from build123d import *

# Parameters (mm, degrees)
BOSS_EXTRUDE1_DEPTH     = 1.5
BOSS_EXTRUDE2_DEPTH     = 280
SKETCH4_W               = 410
SKETCH4_H               = 42.385541564
BOSS_EXTRUDE3_DEPTH     = 30
CUT_EXTRUDE1_DEPTH      = 597.860327045
CUT_EXTRUDE1_DEPTH_BACK = 597.860327045
SKETCH8_R               = 4.39
SKETCH8_R_2             = 2.39
BOSS_EXTRUDE5_DEPTH     = 15
SKETCH10_R              = 3
CUT_EXTRUDE2_DEPTH      = 1.5
SKETCH15_W              = 15
SKETCH15_H              = 1.5
SKETCH15_W_2            = 20
BOSS_EXTRUDE6_DEPTH     = 13
BOSS_EXTRUDE7_DEPTH     = 1.5
BOSS_EXTRUDE8_DEPTH     = 1.5
SKETCH20_R              = 2.415919743
SKETCH20_R_2            = 2
CUT_EXTRUDE5_DEPTH      = 1.5
SKETCH5_R               = 2
SKETCH5_R_2             = 10
CUT_EXTRUDE7_DEPTH      = 1.5
SKETCH21_W              = 300
SKETCH21_H              = 1.5
BOSS_EXTRUDE9_DEPTH     = 10
SKETCH22_W              = 300
SKETCH22_H              = 1.5
BOSS_EXTRUDE10_DEPTH    = 10
BOSS_EXTRUDE11_DEPTH    = 0.75
BOSS_EXTRUDE12_DEPTH    = 0.75
BOSS_EXTRUDE13_DEPTH    = 0.75
BOSS_EXTRUDE14_DEPTH    = 0.75
SKETCH27_W              = 200
SKETCH27_H              = 1.5
BOSS_EXTRUDE15_DEPTH    = 10
BOSS_EXTRUDE16_DEPTH    = 0.75
BOSS_EXTRUDE17_DEPTH    = 0.75
SKETCH30_R              = 24
SKETCH30_R_2            = 1.5
CUT_EXTRUDE8_DEPTH      = 1.5
SKETCH33_R              = 2
CUT_EXTRUDE9_DEPTH      = 1.5


with BuildPart() as part:
    # Sketch1 → Boss-Extrude1 (new body)
    with BuildSketch(Plane(origin=(0, 0, 0), x_dir=(1, 0, 0), z_dir=(0, 1, 0))):
        Polygon((-205, 300), (205, 300), (205, -230), (155, -230), (155, -300), (-205, -300), align=None)
    extrude(amount=BOSS_EXTRUDE1_DEPTH)

    # Sketch2 → Boss-Extrude2 (add)
    with BuildSketch(Plane(origin=(0, 1.5, 0), x_dir=(1, 0, 0), z_dir=(0, 1, 0))):
        Polygon((-205, 300), (-205, -300), (155, -300), (155, -230), (205, -230), (205, 300), align=None)
        Polygon((-203.5, 298.5), (-203.5, -298.5), (153.5, -298.5), (153.5, -228.5), (203.5, -228.5), (203.5, 298.5), align=None, mode=Mode.SUBTRACT)
    extrude(amount=BOSS_EXTRUDE2_DEPTH)

    # Sketch4 → Boss-Extrude3 (add)
    with BuildSketch(Plane(origin=(0, 0, -300), x_dir=(-1, 0, 0), z_dir=(0, 0, -1))):
        with Locations((0, 213.483316708)):
            Rectangle(SKETCH4_W, SKETCH4_H)
    extrude(amount=BOSS_EXTRUDE3_DEPTH)

    # Sketch3 → Cut-Extrude1 (cut, two sides: drawn at the far end of the back side and taken through both)
    with BuildSketch(Plane.ZY.offset(205).offset(-CUT_EXTRUDE1_DEPTH_BACK)):
        Polygon((300, 121.117558148), (228.195222706, 281.5), (300, 281.5), align=None)
    extrude(amount=CUT_EXTRUDE1_DEPTH + CUT_EXTRUDE1_DEPTH_BACK, mode=Mode.SUBTRACT)

    # Sketch8 → Boss-Extrude5 (add)
    # profile 1 of 2: a face of its own
    with BuildSketch(Plane(origin=(-203.5, 0, 0), x_dir=(0, 0, -1), z_dir=(1, 0, 0))):
        with Locations((-261.240414508, 161.097837233)):
            Circle(SKETCH8_R)
        with Locations((-261.240414508, 161.097837233)):
            Circle(SKETCH8_R_2, mode=Mode.SUBTRACT)
    # profile 2 of 2: a face of its own
    with BuildSketch(Plane(origin=(-203.5, 0, 0), x_dir=(0, 0, -1), z_dir=(1, 0, 0))):
        with Locations((-203.5, 16.5)):
            Circle(SKETCH8_R)
        with Locations((-203.5, 16.5)):
            Circle(SKETCH8_R_2, mode=Mode.SUBTRACT)
    extrude(amount=BOSS_EXTRUDE5_DEPTH)

    # Sketch10 → Cut-Extrude2 (cut)
    with BuildSketch(Plane.ZY.offset(-153.5)):
        with BuildLine():
            Line((272.25, 90.5), (258.25, 90.5))
            Line((258.25, 90.5), (258.25, 87.5))
            Line((258.25, 87.5), (254, 87.5))
            ThreePointArc((254, 87.5), (243, 76.5), (254, 65.5))
            Line((254, 65.5), (276.5, 65.5))
            ThreePointArc((276.5, 65.5), (287.5, 76.5), (276.5, 87.5))
            Line((276.5, 87.5), (272.25, 87.5))
            Line((272.25, 87.5), (272.25, 90.5))
        make_face()
        with Locations((239.3, 103.45)):
            Circle(SKETCH10_R)
        with Locations((291.2, 103.45)):
            Circle(SKETCH10_R)
        with Locations((239.3, 49.55)):
            Circle(SKETCH10_R)
        with Locations((291.2, 49.55)):
            Circle(SKETCH10_R)
    extrude(amount=-CUT_EXTRUDE2_DEPTH, mode=Mode.SUBTRACT)

    # Sketch15 → Boss-Extrude6 (add)
    with BuildSketch(Plane.ZY.offset(-203.5)):
        with Locations((-206, 251.386283415)):
            Rectangle(SKETCH15_W, SKETCH15_H)
        with Locations((74.5, 251.386283415)):
            Rectangle(SKETCH15_W_2, SKETCH15_H)
    extrude(amount=BOSS_EXTRUDE6_DEPTH)

    # Sketch17 → Boss-Extrude7 (add)
    with BuildSketch(Plane.XY.offset(-198.5)):
        Polygon((203.5, 250.636283415), (203.5, 235.636283415), (190.5, 250.636283415), align=None)
    extrude(amount=-BOSS_EXTRUDE7_DEPTH)

    # Sketch18 → Boss-Extrude8 (add)
    with BuildSketch(Plane.XY.offset(64.5)):
        Polygon((203.5, 250.636283415), (203.5, 235.636283415), (190.5, 250.636283415), align=None)
    extrude(amount=BOSS_EXTRUDE8_DEPTH)

    # Sketch20 → Cut-Extrude5 (cut)
    with BuildSketch(Plane(origin=(0, 252.136283415, 0), x_dir=(1, 0, 0), z_dir=(0, 1, 0))):
        with Locations(Location((198, 206.5, 0), (0, 0, 270))):
            Circle(SKETCH20_R)
        with Locations(Location((200.5, -77.5, 0), (0, 0, 270))):
            Circle(SKETCH20_R_2)
    extrude(amount=-CUT_EXTRUDE5_DEPTH, mode=Mode.SUBTRACT)

    # Sketch5 → Cut-Extrude7 (cut)
    with BuildSketch(Plane.ZY.offset(205)):
        with Locations((-178.5, 220.666641665)):
            Circle(SKETCH5_R)
        with Locations((-154.5, 196.666641665)):
            Circle(SKETCH5_R)
        with Locations((-154.5, 220.666641665)):
            Circle(SKETCH5_R)
        with Locations((-166.5, 208.666641665)):
            Circle(SKETCH5_R_2)
        with Locations((-178.5, 196.666641665)):
            Circle(SKETCH5_R)
        with Locations((-118.5, 220.666641665)):
            Circle(SKETCH5_R)
        with Locations((-94.5, 196.666641665)):
            Circle(SKETCH5_R)
        with Locations((-94.5, 220.666641665)):
            Circle(SKETCH5_R)
        with Locations((-106.5, 208.666641665)):
            Circle(SKETCH5_R_2)
        with Locations((-118.5, 196.666641665)):
            Circle(SKETCH5_R)
        with Locations((-58.5, 220.666641665)):
            Circle(SKETCH5_R)
        with Locations((-34.5, 196.666641665)):
            Circle(SKETCH5_R)
        with Locations((-34.5, 220.666641665)):
            Circle(SKETCH5_R)
        with Locations((-46.5, 208.666641665)):
            Circle(SKETCH5_R_2)
        with Locations((-58.5, 196.666641665)):
            Circle(SKETCH5_R)
        with Locations((1.5, 220.666641665)):
            Circle(SKETCH5_R)
        with Locations((25.5, 196.666641665)):
            Circle(SKETCH5_R)
        with Locations((25.5, 220.666641665)):
            Circle(SKETCH5_R)
        with Locations((13.5, 208.666641665)):
            Circle(SKETCH5_R_2)
        with Locations((1.5, 196.666641665)):
            Circle(SKETCH5_R)
    extrude(amount=-CUT_EXTRUDE7_DEPTH, mode=Mode.SUBTRACT)

    # Sketch21 → Boss-Extrude9 (add)
    with BuildSketch(Plane(origin=(0, 0, -300), x_dir=(-1, 0, 0), z_dir=(0, 0, -1))):
        with Locations((0, 270.75)):
            Rectangle(SKETCH21_W, SKETCH21_H)
    extrude(amount=BOSS_EXTRUDE9_DEPTH)

    # Sketch22 → Boss-Extrude10 (add)
    with BuildSketch(Plane.ZY.offset(205)):
        with Locations((-70, 270.75)):
            Rectangle(SKETCH22_W, SKETCH22_H)
    boss_extrude10 = extrude(amount=BOSS_EXTRUDE10_DEPTH)

    # Sketch23 → Boss-Extrude11 (add, symmetric)
    with BuildSketch(Plane(origin=(0, 0, -140), x_dir=(-1, 0, 0), z_dir=(0, 0, -1))):
        Polygon((215, 270), (205, 270), (205, 260), align=None)
    boss_extrude11 = extrude(amount=BOSS_EXTRUDE11_DEPTH, both=True)

    # Sketch24 → Boss-Extrude12 (add, symmetric)
    with BuildSketch(Plane.XY.offset(-10)):
        Polygon((-215, 270), (-205, 260), (-205, 270), align=None)
    boss_extrude12 = extrude(amount=BOSS_EXTRUDE12_DEPTH, both=True)

    # Sketch25 → Boss-Extrude13 (add, symmetric)
    with BuildSketch(Plane(origin=(100, 0, 0), x_dir=(0, 0, -1), z_dir=(1, 0, 0))):
        Polygon((310, 270), (300, 270), (300, 260), align=None)
    extrude(amount=BOSS_EXTRUDE13_DEPTH, both=True)

    # Sketch26 → Boss-Extrude14 (add, symmetric)
    with BuildSketch(Plane.ZY.offset(100)):
        Polygon((-310, 270), (-300, 260), (-300, 270), align=None)
    extrude(amount=BOSS_EXTRUDE14_DEPTH, both=True)

    # Mirror1: Boss-Extrude10, Boss-Extrude11, Boss-Extrude12 across plane
    add(boss_extrude10.mirror(Plane(origin=(0, 0, 0), x_dir=(0, 0, 1), z_dir=(1, 0, 0))))
    add(boss_extrude11.mirror(Plane(origin=(0, 0, 0), x_dir=(0, 0, 1), z_dir=(1, 0, 0))))
    add(boss_extrude12.mirror(Plane(origin=(0, 0, 0), x_dir=(0, 0, 1), z_dir=(1, 0, 0))))

    # Sketch27 → Boss-Extrude15 (add)
    with BuildSketch(Plane.XY.offset(300)):
        with Locations((-25, 110.367558148)):
            Rectangle(SKETCH27_W, SKETCH27_H)
    extrude(amount=BOSS_EXTRUDE15_DEPTH)

    # Sketch28 → Boss-Extrude16 (add, symmetric)
    with BuildSketch(Plane.ZY.offset(95)):
        Polygon((310, 109.617558148), (300, 109.617558148), (300, 99.617558148), align=None)
    extrude(amount=BOSS_EXTRUDE16_DEPTH, both=True)

    # Sketch29 → Boss-Extrude17 (add, symmetric)
    with BuildSketch(Plane(origin=(45, 0, 0), x_dir=(0, 0, -1), z_dir=(1, 0, 0))):
        Polygon((-310, 109.617558148), (-300, 99.617558148), (-300, 109.617558148), align=None)
    extrude(amount=BOSS_EXTRUDE17_DEPTH, both=True)

    # Sketch30 → Cut-Extrude8 (cut)
    with BuildSketch(Plane(origin=(205, 0, 0), x_dir=(0, 0, -1), z_dir=(1, 0, 0))):
        with Locations((-196.5, 160)):
            Circle(SKETCH30_R)
        with Locations((-222.5, 150)):
            Circle(SKETCH30_R_2)
        with Locations((-170.5, 150)):
            Circle(SKETCH30_R_2)
    extrude(amount=-CUT_EXTRUDE8_DEPTH, mode=Mode.SUBTRACT)

    # Sketch33 → Cut-Extrude9 (cut)
    with BuildSketch(Plane.ZY.offset(205)):
        with Locations((-242.8, 147.77)):
            Circle(SKETCH33_R)
        with Locations((-242.8, 28.39)):
            Circle(SKETCH33_R)
        with Locations((-71.1, 147.77)):
            Circle(SKETCH33_R)
        with Locations((-71.1, 28.39)):
            Circle(SKETCH33_R)
        with Locations((100.6, 147.77)):
            Circle(SKETCH33_R)
        with Locations((100.6, 28.39)):
            Circle(SKETCH33_R)
    extrude(amount=-CUT_EXTRUDE9_DEPTH, mode=Mode.SUBTRACT)


solid = part.part
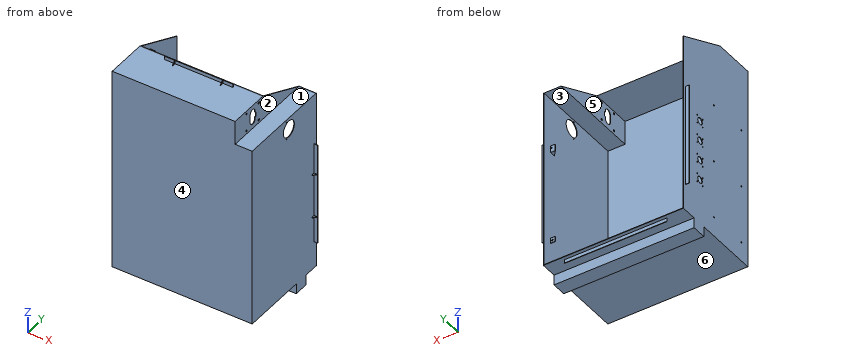
Read the model definition and answer for the solid it produces. Units are mm, in the model's axes. Face numbers are marked on the shaded views. A direction names the side the tool comes from. Round coordinates to 2 decimals unless told otherwise and drop trailing zeros. Write each loop counter-clockwise with the first axis right and the second up, starting at its lowest first coordinate (ties: lowest second). Pieces come first, ordered by that corner, then holes.
Q1. Find section D-D on z = 126. Determine the outline of the cut face in (x, y).
Values:
outline: (-205, 0) - (205, 0) - (205, 281.5) - (203.5, 281.5) - (203.5, 1.5) - (-203.5, 1.5) - (-203.5, 281.5) - (-205, 281.5) - close
Q2. Straight lines are drawn through the part: line 1 (Y direction, x = -203.8, z = -154.5); line 2 (Y direction, x = -204, z = 100); line 3 (Z direction, x = 200.5, y = 251.05). For each, find the intervals that lie inside material, in ascending order.
Values:
line 1: y = 0 to 194.67, 198.67 to 218.67, 222.67 to 281.5
line 2: y = 0 to 26.48, 30.3 to 145.86, 149.68 to 281.5
line 3: z = -300 to -298.5, -213.5 to -198.5, 64.5 to 75.5, 79.5 to 84.5, 228.5 to 230
Q3. Find section B-B on y = 76.5. Determine the outline of the cut face in (x, z).
Values:
outline: (-205, -300) - (205, -300) - (205, 230) - (155, 230) - (155, 243) - (153.5, 243) - (153.5, 228.5) - (203.5, 228.5) - (203.5, -298.5) - (-203.5, -298.5) - (-203.5, 298.5) - (153.5, 298.5) - (153.5, 287.5) - (155, 287.5) - (155, 300) - (-205, 300) - close
Q4. A tool of negligible diameter and unlimited length cuts with its end or side. For the marked faces 4, 5 and 6, from which of +Z, -Z, +X, -X, +Y, -Y can it reach the whole face along a straight path? Write none if from no direction.
Values:
face 4: +Z, -Z, +X, -X, -Y
face 5: +Y
face 6: -Z, +X, -X, -Y
Q5. The mould has two halves that part along X. Classify the marked faces 1, 2 and 3: released by +X, released by -X, zero draft, split by the parting line, or undercut.
Values:
face 1: zero draft
face 2: released by +X
face 3: undercut
Q6. Find section C-C on x = -45. Determine the outline of the cut face in (y, z), and give its area (3 significant figures).
Values:
outline: (0, -300) - (192.29, -300) - (192.29, -330) - (234.68, -330) - (234.68, -300) - (270, -300) - (270, -310) - (271.5, -310) - (271.5, -300) - (281.5, -300) - (281.5, -298.5) - (1.5, -298.5) - (1.5, 298.5) - (124.47, 298.5) - (121.12, 300) - (111.12, 300) - (111.12, 310) - (109.62, 310) - (109.62, 300) - (0, 300) - close
area: 2,800 mm2
Q7. Flat-ended cylindrical pins translate along their axes: P1, Ø5.5, axis at y = 161.5, z = 261, coming from the +X side; P2, Ø10, axis at y = 84, z = 230, coming from the +X side; P3, Ø1.6, axis at x = 154, z = 264.5, coming from the -Y side; P4, Ø6, axis at x = 156, y = 221, coming from the +Z side. Find the tip coordinate at first contact, or state that the pin passes through.
Values:
P1: stops at x = 155
P2: stops at x = 205
P3: stops at y = 0
P4: stops at z = 256.55
Q8. Find section A-A on z = 13.5. Determine the outline of the cut face in (x, y), and give its area (4 significant figures).
Values:
outline: (-215, 270) - (-205, 270) - (-205, 218.67) - (-203.5, 218.67) - (-203.5, 281.5) - (-205, 281.5) - (-205, 271.5) - (-215, 271.5) - close; (-205, 0) - (205, 0) - (205, 270) - (215, 270) - (215, 271.5) - (205, 271.5) - (205, 281.5) - (203.5, 281.5) - (203.5, 1.5) - (-203.5, 1.5) - (-203.5, 198.67) - (-205, 198.67) - close
area: 1,455 mm2
